CAD build for the part. Positions are in the model's coordinates, mm. Face numbers are marked on the shaded views. Round coordinates to 2 decimals unless told otherwise and drop trailing zeros. Order: outer loops, then holes, each group sorted by start corner. A loop starts at its lowest first (then second) coordinate and runs counter-clockwise, first axis right, second up. Notation, with made-up numbers: M 28,5.5 L 42,5.5 A16 cw 42,9.5 Z; hole C -27.5,5.5 d5. An arc over 180 degrees is marked long. Answer as a JSON object with one key per item and string values.
```python
from build123d import *

# Parameters (mm, degrees)
F0_R     = 9.25
F0_R_2   = 7
F1_DEPTH = 40
F2_R     = 7.5
F4_DEPTH = 2
F5_R     = 7.75
F5_R_2   = 7
F6_DEPTH = 4


# Not quite as in the source:
# - a fillet or chamfer that OpenCascade refuses, or shapes differently, is made with other operations: its cross-section is extruded or revolved along the edge and cut away or added


with BuildPart() as f1:
    # F0 (on Top) → F1 (new body)
    with BuildSketch(Plane.XY):
        Circle(F0_R)
        Circle(F0_R_2, mode=Mode.SUBTRACT)
    extrude(amount=F1_DEPTH)

    # F3: fillet of radius 3 on 1 edges, made by hand

    # F3_s1 → F3_t2 (revolve, cut)
    with BuildSketch(Plane.XZ):
        with BuildLine():
            ThreePointArc((9.25, 2.9047375097), (8.6217082451, 1.0676202026), (7, 0))
            Line((7, 0), (9.25, 0))
            Line((9.25, 0), (9.25, 2.9047375097))
        make_face()
    revolve(axis=Axis((0, 0, 0), (0, 0, 1)), mode=Mode.SUBTRACT)

    # F2 (on face) → F4 (join)
    with BuildSketch(Plane(origin=(0, 0, 0), x_dir=(1, 0, 0), z_dir=(0, 0, -1))):
        Circle(F2_R)
    extrude(amount=-F4_DEPTH)

    # F5 (on face) → F6 (join)
    with BuildSketch(Plane.XY.offset(40)):
        Circle(F5_R)
        Circle(F5_R_2, mode=Mode.SUBTRACT)
    extrude(amount=F6_DEPTH)


solid = f1.part
```
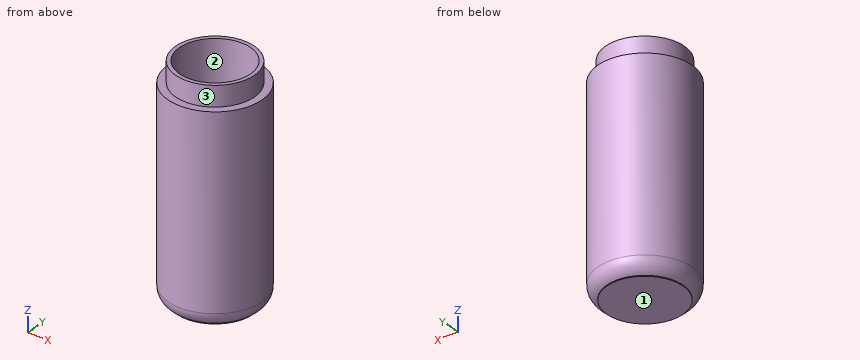
Item 1: Drop flat-ended pins along their axis: pin 1 Ø3 at (x, z) = (-5.5, 27) entering from +Y; pin 2 Ø4 at (x, z) = (3, 24.5) entering from -Y; pin 3 Ø6 at (x, y) = (-1, 2) entering from +Z. Give the stop position or say it passes through.
Worked answers:
{"pin 1": "stops at y = 8.34", "pin 2": "stops at y = -9.2", "pin 3": "stops at z = 2"}
Item 2: Saw through at C-C on z = 20. List the corners of the cut face in (x, y), and give its area (3 significant figures).
Worked answers:
{"outline": "C 0,0 d18.5; hole C 0,0 d14", "area": "115 mm2"}
Item 3: Wall check: line 1 along Y through (x, z) = (0, 24.5); line 2 along X through (y, z) = (-5.75, 34.5). Give the ranges that are in metal, low to high. Write a range as [from, to].
Worked answers:
{"line 1": "y = [-9.25, -7], [7, 9.25]", "line 2": "x = [-7.25, -3.99], [3.99, 7.25]"}
Item 4: Two-plate mould, pull along X, no slides. Class the marked faces 1, 2 and 3: released by +X, released by -X, zero draft, split by the parting line, or undercut.
Worked answers:
{"face 1": "zero draft", "face 2": "undercut", "face 3": "split by the parting line"}
Item 5: Saw through at A-A on y = 0. List the corners of the cut face in (x, z).
Worked answers:
{"outline": "M -9.25,2.9 A3 ccw -7.5,0.18 L -7.5,0 L 7.5,0 L 7.5,0.18 A3 ccw 9.25,2.9 L 9.25,40 L 7.75,40 L 7.75,44 L 7,44 L 7,2 L -7,2 L -7,44 L -7.75,44 L -7.75,40 L -9.25,40 Z"}
